Design review of the part shown in the three views and the two pictorial views. Dimensions are in mm from the part's minimum x, y and z. Coordinates: 2 decimals unless noted, no trailing zeros. Order: outer loops, then holes, each group sorted by start corner. A loop starts at its lowest first (then second) coordinate and runs counter-clockwise, first axis right, second up. Notation, with made-up numbers: (8, 71) -> (45, 71) arc R24 cw to (45, 85) -> close; hole circle Ø11 at (64, 86). An arc over 180 degrees is marked (long way). Answer as a JSON object with one key per item and string values. Group by question number.
1) For pin 1 (2 mm diameter, centred on y = 3.5, z = 2.5, fed in from -X); pin 2 (2 mm diameter, centred on x = 4.5, z = 4, fed in from -Y), all flat-tipped, find the tip position at first contact; note any pin that passes through.
2) Wall thickness on L1, parallel to Y at x = 2.25, z = 8.75; L2, parallel to X at y = 1.9, z = 4 (1 decimal); L3, parallel to X at y = 3.15, z = 4: over which ranges is each line inside the solid? List them lowest first.
3) Add section C-C, the plane x = 5.2. Write out the cut boundary in (y, z).
4) Draft analysis for pull direction Y (two halves, no side actions). For the marked faces 1, 2, 3 and 4, state which applies: +Y half, -Y half, draft (parallel to the pull), parting line (faces both ways), or undercut.
5) Add section D-D, the plane x = 4.6. Write out the cut boundary in (y, z).
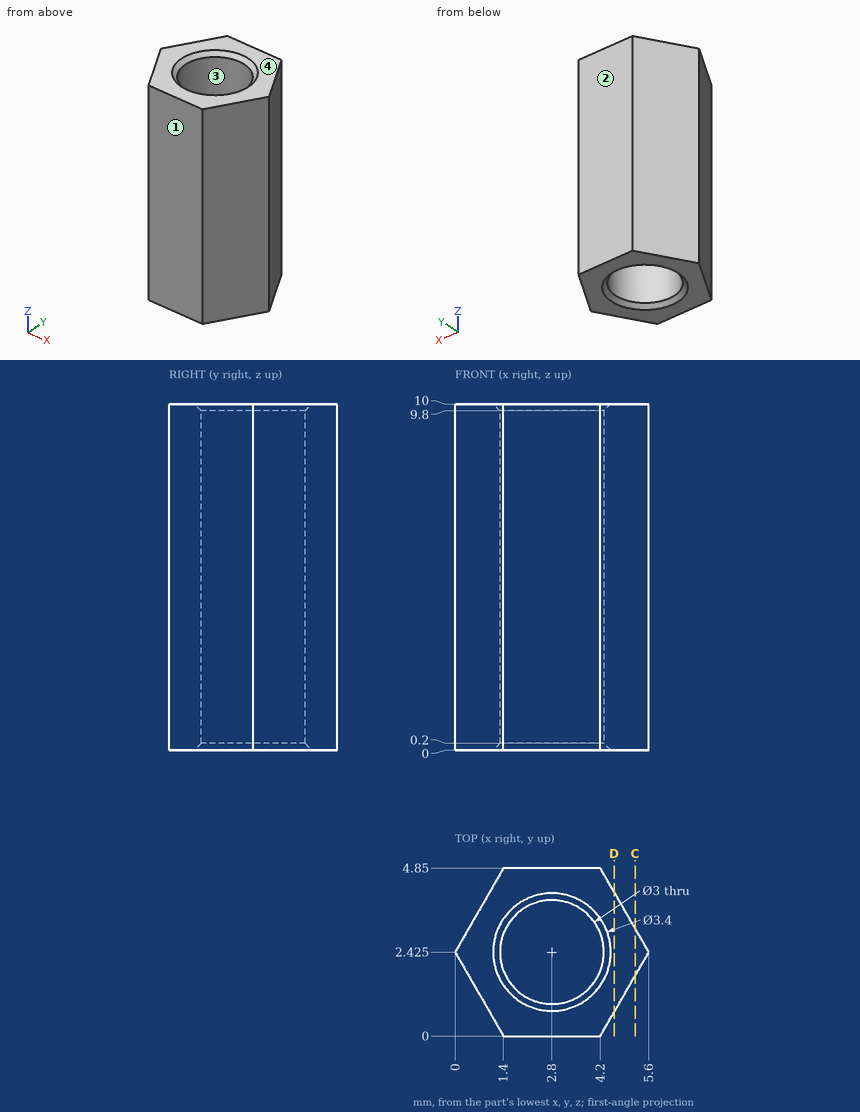
Output values:
{
 "1": {"pin 1": "stops at x = 0.04", "pin 2": "stops at y = 0"},
 "2": {"L1": "y = 0 to 1.03, 3.82 to 4.85", "L2": "x = 0.3 to 1.4, 4.2 to 5.3", "L3": "x = 0.42 to 1.49, 4.11 to 5.18"},
 "3": {"outline": "(1.73, 0) -> (3.12, 0) -> (3.12, 10) -> (1.73, 10) -> close"},
 "4": {"face 1": "-Y half", "face 2": "+Y half", "face 3": "undercut", "face 4": "draft"},
 "5": {"outline": "(0.69, 0) -> (4.16, 0) -> (4.16, 10) -> (0.69, 10) -> close"}
}
